Verification items for the finished model (mm, model axes). A direction names the side the tool comes from. Give positions to 0.01 mm unless a question says otherwise; leave off trailing zeros. Write each loop counter-clockwise with the first axis right and the second up, starting at its lowest first coordinate (ties: lowest second). Pieces come first, ordered by that corner, then holes.
from build123d import *

# Parameters (mm, degrees)
ESQUISSE1_R             = 35.5
BOSS_EXTRU_1_DEPTH      = 20
CONG_1_R                = 3
ESQUISSE2_R             = 4
ENL_V_MAT_EXTRU_1_DEPTH = 2


# Read off the part's stored shape, not the designer's step: Coque1
with BuildPart() as part:
    # Esquisse1 → Boss.-Extru.1 (new body)
    with BuildSketch(Plane(origin=(0, 0, 0), x_dir=(1, 0, 0), z_dir=(0, 1, 0))):
        with Locations(Location((0, 0, 0), (0, 0, 270))):
            Circle(ESQUISSE1_R)
    extrude(amount=BOSS_EXTRU_1_DEPTH)

    # Congé1
    cong_1_edges = [part.edges().sort_by_distance(p)[0] for p in [
        (0, 20, -35.5),
    ]]
    fillet(cong_1_edges, radius=CONG_1_R)

    # Coque1 outline → Coque1 (revolve, cut)
    with BuildSketch(Plane.XY):
        with BuildLine():
            Line((34.5, 0), (34.5, 17))
            ThreePointArc((34.5, 17), (33.914213562, 18.414213562), (32.5, 19))
            Line((32.5, 19), (0, 19))
            Line((0, 19), (0, 0))
            Line((0, 0), (34.5, 0))
        make_face()
    revolve(axis=Axis((0, 0, 0), (0, 1, 0)), mode=Mode.SUBTRACT)

    # Esquisse2 → Enlèv. mat.-Extru.1 (cut)
    with BuildSketch(Plane(origin=(0, 20, 0), x_dir=(1, 0, 0), z_dir=(0, 1, 0))):
        with Locations(Location((0, 0, 0), (0, 0, 270))):
            Circle(ESQUISSE2_R)
    extrude(amount=-ENL_V_MAT_EXTRU_1_DEPTH, mode=Mode.SUBTRACT)


solid = part.part
Item 1: Set-up check for faces 4 (the face through (7, 19, 0)), 5 (the face through (19, 0, -29)): record each of +Z, -Z, +X, -X, +Y, -Y from which the full face is reachable in a straight line by a thin tool's end or side.
Answer key:
face 4: -Y
face 5: +Z, -Z, +X, -X, -Y
Item 2: Sectioned sample at B-B on z = 0. Record the cut outline in (x, y).
Answer key:
outline: (-35.5, 0) - (-34.5, 0) - (-34.5, 17) arc R2 cw to (-32.5, 19) - (-4, 19) - (-4, 20) - (-32.5, 20) arc R3 ccw to (-35.5, 17) - close; (4, 19) - (32.5, 19) arc R2 cw to (34.5, 17) - (34.5, 0) - (35.5, 0) - (35.5, 17) arc R3 ccw to (32.5, 20) - (4, 20) - close
Item 3: Sectioned sample at A-A on x = 0. Record the cut outline in (y, z).
Answer key:
outline: (0, -35.5) - (17, -35.5) arc R3 ccw to (20, -32.5) - (20, -4) - (19, -4) - (19, -32.5) arc R2 cw to (17, -34.5) - (0, -34.5) - close; (0, 34.5) - (17, 34.5) arc R2 cw to (19, 32.5) - (19, 4) - (20, 4) - (20, 32.5) arc R3 ccw to (17, 35.5) - (0, 35.5) - close
Item 4: Release check for a two-part mould opening along X. For faces 1 (the face through (0, 20, 7)), 2 (the face through (-31.495, 8.381, 16.381)), 3 (the face through (32.907, 8.619, -10.363)) record: released by +X, released by -X, zero draft, split by the parting line, or undercut.
Answer key:
face 1: zero draft
face 2: split by the parting line
face 3: undercut
Item 5: Sectioned sample at C-C on y = 13.25. Record the cut outline in (x, z), then the cut area to 3 significant figures.
Answer key:
outline: circle Ø71 at (0, 0); hole circle Ø69 at (0, 0)
area: 220 mm2
Item 6: Scan lines: line 1 along X through (y, z) = (3.5, 0); line 2 along X through (y, z) = (2, 7); line 3 along Y through (x, z) = (-16, 2.5). Record each from-to range of solid material in increasing order.
Answer key:
line 1: x = -35.5 to -34.5, 34.5 to 35.5
line 2: x = -34.8 to -33.78, 33.78 to 34.8
line 3: y = 19 to 20
Item 7: Depth check by flat-ended pin: pin 1 (6 mm diameter, centred on y = 4, z = 12.5, fed in from +X); pin 2 (1 mm diameter, centred on y = 14, z = -7.5, fed in from +X); pin 3 (1.5 mm diameter, centred on y = 13.5, z = 17.5, fed in from -X). Enter the tip coordinate at first touch or a pass-through.
Answer key:
pin 1: stops at x = 34.21
pin 2: stops at x = 34.8
pin 3: stops at x = -31.3
